Design review of the part built by this model. Coordinates are the model's own, in mm. Round coordinates to 2 decimals unless told otherwise and drop trailing zeros. Order: outer loops, then holes, each group sorted by start corner. A loop starts at its lowest first (then second) coordinate and runs counter-clockwise, first axis right, second up. Notation, with made-up numbers: (-15, 46) - (8, 46) arc R9 cw to (8, 62) - close; hole circle Ø5 at (-36.75, 84.5). An arc over 180 degrees is marked (long way). Write item = value, one per line.
from build123d import *

# Parameters (mm, degrees)
SKETCH1_R            = 84
SKETCH1_R_2          = 45
BOSS_EXTRUDE1_DEPTH  = 10
M6_CLEARANCE_HOLE1_D = 7


with BuildPart() as part:
    # Sketch1 → Boss-Extrude1 (new body)
    with BuildSketch(Plane(origin=(0, 0, 0), x_dir=(1, 0, 0), z_dir=(0, 1, 0))):
        with Locations(Location((0, 0, 0), (0, 0, 270))):
            Circle(SKETCH1_R)
        with Locations(Location((0, 0, 0), (0, 0, 270))):
            Circle(SKETCH1_R_2, mode=Mode.SUBTRACT)
    extrude(amount=BOSS_EXTRUDE1_DEPTH)

    # M6 Clearance Hole1 (through all)
    with Locations(Plane(origin=(-76, 10, 0), x_dir=(0, 0, 1), z_dir=(0, 1, 0))):
        with Locations((0, 0), (-76, 76), (0, 152), (76, 76)):
            Hole(M6_CLEARANCE_HOLE1_D / 2)


solid = part.part
1) To check wall thickness, follow L1, parallel to X at y = 7.5, z = 0; L2, parallel to Z at x = -27, y = 5.25; L3, parallel to Z at x = -3, y = 9.5. State the ranges of each line that lie inside material, in increasing order. Write a range as from..to.
Findings:
L1 = -84..-79.5, -72.5..-45, 45..72.5, 79.5..84
L2 = -79.54..-36, 36..79.54
L3 = -83.95..-77.8, -74.2..-44.9, 44.9..74.2, 77.8..83.95
2) We need section A-A on x = 0. Write out the cut boundary in (y, z).
Findings:
outline = (0, -84) - (10, -84) - (10, -79.5) - (0, -79.5) - close; (0, -72.5) - (10, -72.5) - (10, -45) - (0, -45) - close; (0, 45) - (10, 45) - (10, 72.5) - (0, 72.5) - close; (0, 79.5) - (10, 79.5) - (10, 84) - (0, 84) - close
3) We need section D-D on x = 23. Write out the cut boundary in (y, z).
Findings:
outline = (0, -80.79) - (10, -80.79) - (10, -38.68) - (0, -38.68) - close; (0, 38.68) - (10, 38.68) - (10, 80.79) - (0, 80.79) - close
4) We need section B-B on z = -29. Write out the cut boundary in (x, y).
Findings:
outline = (-78.84, 0) - (-34.41, 0) - (-34.41, 10) - (-78.84, 10) - close; (34.41, 0) - (78.84, 0) - (78.84, 10) - (34.41, 10) - close
5) The part is to be moulded in two halves that separate along Z. For faces 1 (the cylindrical face through (25.23, 4.93, 80.12)), 2 (the flat face through (-36, 0, 36)), 3 (the cylindrical face through (-17.235, 4.93, 41.569)), say which applies: released by +Z, released by -Z, zero draft, split by the parting line, or undercut.
Findings:
face_1 = split by the parting line
face_2 = zero draft
face_3 = undercut
6) Clearance check with flat-ended pins moving along their axes: pin 1 Ø3 at (y, z) = (2.5, 35) entering from +X; pin 2 Ø1.5 at (x, y) = (-5, 2) entering from +Z; pin 3 Ø6.5 at (x, z) = (0, 76) entering from -Y; pin 4 Ø1.5 at (y, z) = (4.5, 28.5) entering from +X. State where each tip first meets the part, or that it passes through.
Findings:
pin_1 = 77.03
pin_2 = 83.89
pin_3 = through
pin_4 = 79.28
7) We need section C-C on y = 5. Write out the cut boundary in (x, z), and give its area (3 significant figures).
Findings:
outline = circle Ø168 at (0, 0); hole circle Ø7 at (-76, 0); hole circle Ø90 at (0, 0); hole circle Ø7 at (0, -76); hole circle Ø7 at (0, 76); hole circle Ø7 at (76, 0)
area = 15,700 mm^2
